Input: part model. Units: mm. Frame: model coordinates. Face numbers are marked on the shaded views. A direction names the side the tool comes from. Round coordinates to 2 decimals unless told otherwise and drop trailing zeros. Order: outer loops, then holes, each group sorted by start corner. A loop starts at its lowest first (then second) coordinate and runs counter-clockwise, first axis right, second up. Notation, with made-up numbers: M 26.25,-25 L 84.25,-25 A26 cw 84.25,14 Z; hole C 76.25,73.5 d10. An arc over 180 degrees is marked long. One line per question, with ' | ' between items.
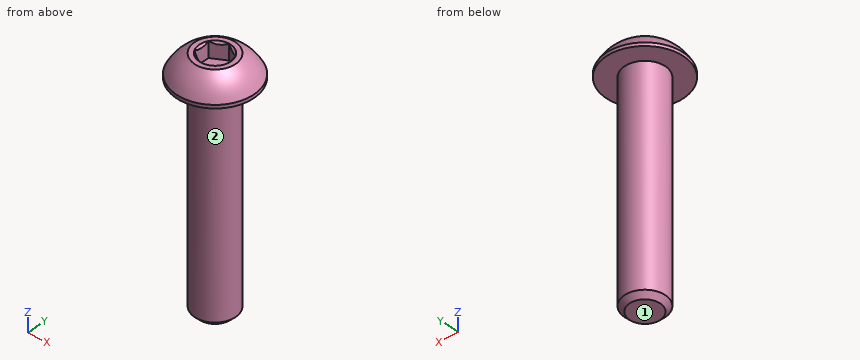
```python
from build123d import *

# Parameters (mm, degrees)
CUT_EXTRUDE2_DEPTH = 1.155


with BuildPart() as part:
    # Sketch10 → Revolve3 (revolve)
    with BuildSketch(Plane(origin=(0, 0, 0), x_dir=(0, 0, -1), z_dir=(1, 0, 0)), mode=Mode.PRIVATE) as revolve3_sk:
        Polygon((7.625, 1.5), (8, 1.125), (8, 0), (-8, 0), (-8, 1.5), align=None)
    revolve(revolve3_sk.sketch.rotate(Axis((0, 0, 9.65), (0, 0, -1)), 180), axis=Axis((0, 0, 9.65), (0, 0, -1)))

    # Sketch7 → Revolve2 (revolve)
    with BuildSketch(Plane(origin=(0, 0, 0), x_dir=(0, 0, -1), z_dir=(1, 0, 0)), mode=Mode.PRIVATE) as revolve2_sk:
        with BuildLine():
            Line((-8.2475, 2.85), (-8, 2.85))
            Line((-8, 2.85), (-8, 0))
            Line((-8, 0), (-9.65, 0))
            Line((-9.65, 0), (-9.65, 1.5))
            ThreePointArc((-9.65, 1.5), (-9.05487489, 2.285251969), (-8.2475, 2.85))
        make_face()
    revolve(revolve2_sk.sketch.rotate(Axis((0, 0, 9.65), (0, 0, -1)), 180), axis=Axis((0, 0, 9.65), (0, 0, -1)))

    # Sketch5 → Cut-Extrude2 (cut)
    with BuildSketch(Plane.XY.offset(9.65)):
        Polygon((1, -0.577350269), (1, 0.577350269), (0, 1.154700538), (-1, 0.577350269), (-1, -0.577350269), (0, -1.154700538), align=None)
    extrude(amount=-CUT_EXTRUDE2_DEPTH, mode=Mode.SUBTRACT)

    # Cut-Extrude3 cone 1 section (on through the dimple's axis) → Cut-Extrude3 (revolve, cut)
    with BuildSketch(Plane(origin=(0, 0, 9.65), x_dir=(0, -1, 0), z_dir=(1, 0, 0))):
        Polygon((0, 0), (1.154700538, 0), (0, 1.154700538), align=None)
    revolve(axis=Axis((0, 0, 9.65), (0, 0, -1)), mode=Mode.SUBTRACT)


solid = part.part
```
Item 1: Access query for the marked faces 1 and 2. Directions: +Z, -Z, +X, -X, +Y, -Y. A direction counts if a zero-diameter tool reaches every point of the face in a straight line with its end or side. Return the directions, or none.
Report:
face 1: -Z, +X, -X, +Y, -Y | face 2: -Z
Item 2: First-contact query: pin 1 (1 mm diameter, centred on x = 0, y = -0.5, fed in from +Z) (3 decimals); pin 2 (2 mm diameter, centred on y = -0.5, z = 5, fed in from -X); pin 3 (1.3 mm diameter, centred on y = 0, z = 9, fed in from -X). Flat tips, straight axial feed; report the tip coordinate or a pass-through.
Report:
pin 1: z = 8.495 | pin 2: x = -1.5 | pin 3: x = -2.8
Item 3: Section query B-B, the plane z = 5. Return loops of the section in (x, y), plus the area to 3 significant figures.
Report:
outline: C 0,0 d3 | area: 7.07 mm²
Item 4: Section query C-C, the plane x = 1.8. Return loops of the section in (y, z).
Report:
outline: M -2.21,8 L 2.21,8 L 2.21,8.25 A2.61 ccw -2.21,8.25 Z
Item 5: Line query: line 1 along Z through (x, y) = (0, -0.95) (3 decimals); line 2 along Y through (x, z) = (-0.6, 5.5); line 3 along X through (y, z) = (-1.1, 7.5). Output: solid intervals per line, ascending. Write a range as from..to.
Report:
line 1: -8..8.495 | line 2: -1.37..1.37 | line 3: -1.02..1.02
Item 6: Section query D-D, the plane y = 2.1. Return loops of the section in (x, z).
Report:
outline: M -1.93,8 L 1.93,8 L 1.93,8.25 A2.38 ccw -1.93,8.25 Z
